Work out the finished part from the listing and answer in its coordinate system (mm). Face numbers are marked on the shaded views. A direction names the side the tool comes from. Coordinates: 2 decimals unless noted, no trailing zeros. Write each loop counter-clockwise with the first axis right and the second up, starting at its lowest first coordinate (ties: lowest second). Pieces come first, ordered by that corner, then holes. Notation, with made-up numbers: M 87,36.25 L 127,36.25 A14 ccw 127,56.25 Z; hole C -35,-14.75 d6. An arc over 180 degrees is marked long. Answer as CSV lines item,"result". Start each with the question number.
(1) Flat-ended cylindrical pins translate along their axes: P1, Ø3.5, axis at x = -243.73, y = 56.34, coming from the -Z side; P2, Ø4, axis at x = -194, z = 7.5, coming from the +Y side; P3, Ø3, axis at x = -229, z = 2.5, coming from the +Y side. Find the tip coordinate at first contact, or state that the pin passes through.
(2) The mould has two halves that part along X. Classify the marked faces 3, 4, 5 and 6: released by +X, released by -X, zero draft, split by the parting line, or undercut.
(3) Find the intervals of material crossed by L1, parallel to X at y = 53, z = 11; L2, parallel to Y at x = -185, z = 6.5; L3, parallel to X at y = 64, z = 8.25, in increasing order. Write a range as [from, to].
(4) For the marked faces 1 and 2, determine the directions among +Z, -Z, +X, -X, +Y, -Y from which every point of the face is accessible in a straight line to the end or side of a thin tool.
(5) A cutting plane is placed at B-B on z = 11. Count the separate pieces of the cut face and the enclosed holes in it, then the cut area to 3 significant figures.
(6) A cutting plane is placed at A-A on y = 2. Give the vertices of the cut face in (x, z).
(7) A cutting plane is placed at C-C on x = -179.5. Give the vertices of the cut face in (y, z).
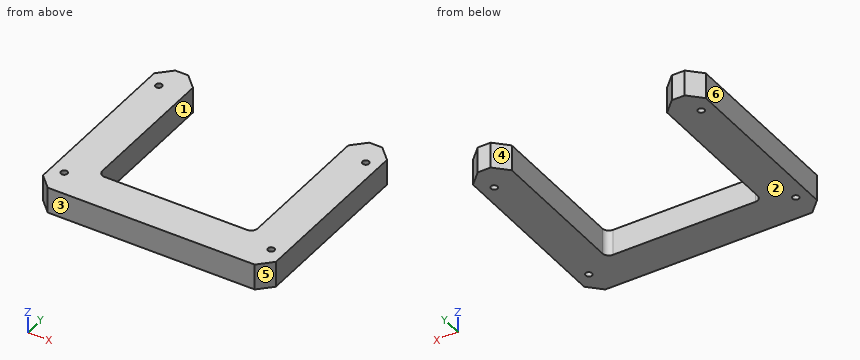
from build123d import *

# Parameters (mm, degrees)
BOSS_EXTRUDE1_DEPTH = 12.7
FILLET1_R           = 3.175
CHAMFER1_SIZE       = 6.35
HOLE1_D             = 3.175
HOLE1_DEPTH         = 31.75
HOLE1_CSINK_D       = 10.16
HOLE1_CSINK_ANGLE   = 82
HOLE1_TIP           = 0.953866233


with BuildPart() as part:
    # Sketch1 → Boss-Extrude1 (new body)
    with BuildSketch(Plane.XY):
        Polygon((-231.027465963, 69.04320968), (-231.027465963, -10.33179032), (-154.827465963, -10.33179032), (-154.827465963, 69.04320968), (-135.777465963, 69.04320968), (-135.777465963, -29.38179032), (-250.077465963, -29.38179032), (-250.077465963, 69.04320968), align=None)
    extrude(amount=BOSS_EXTRUDE1_DEPTH)

    # Fillet1
    fillet1_edges = [part.edges().sort_by_distance(p)[0] for p in [
        (-231.027465963, -10.33179032, 6.35),
        (-154.827465963, -10.33179032, 6.35),
    ]]
    fillet(fillet1_edges, radius=FILLET1_R)

    # Chamfer1
    chamfer1_edges = [part.edges().sort_by_distance(p)[0] for p in [
        (-231.027465963, 69.04320968, 6.35),
        (-154.827465963, 69.04320968, 6.35),
        (-135.777465963, 69.04320968, 6.35),
        (-135.777465963, -29.38179032, 6.35),
        (-250.077465963, -29.38179032, 6.35),
        (-250.077465963, 69.04320968, 6.35),
    ]]
    chamfer(chamfer1_edges, length=CHAMFER1_SIZE)

    # Hole1
    with Locations(Plane(origin=(-124.004465969, -215.287141225, -12.7), x_dir=(-1, 0, 0), z_dir=(0, 0, -1))):
        with Locations((113.649999994, 128.807623392), (113.649999994, 23.940956725), (-94.599999994, 161.374290059), (94.599999994, 161.374290059), (0, 161.374290059), (0, 193.124290059), (0, 440.553783621), (0, 301.970350905), (40.979166666, 301.970350905), (166.795833328, 301.970350905), (207.774999994, 440.553783621), (207.774999994, 333.02141023), (207.774999994, 225.48903684), (207.774999994, 137.424290059), (207.774999994, 10.424290059), (-207.774999994, 10.424290059), (-207.774999994, 137.424290059), (-207.774999994, 225.48903684), (-207.774999994, 333.02141023), (-207.774999994, 440.553783621), (-166.795833328, 301.970350905), (-40.979166666, 301.970350905), (-113.649999994, 23.940956725), (-113.649999994, 128.807623392), (119.722999994, 198.605350905), (119.722999994, 271.630350905), (18.122999994, 198.605350905), (18.122999994, 271.630350905)):
            CounterSinkHole(HOLE1_D / 2, HOLE1_CSINK_D / 2, depth=HOLE1_DEPTH, counter_sink_angle=HOLE1_CSINK_ANGLE)
            with Locations((0, 0, -(HOLE1_DEPTH + HOLE1_TIP / 2))):  # 118° drill point
                Cone(0, HOLE1_D / 2, HOLE1_TIP, mode=Mode.SUBTRACT)


solid = part.part
Here are the results:
1,P1,"stops at z = 0"
1,P2,"stops at y = -10.33"
1,P3,"stops at y = -8.91"
2,face 3,"zero draft"
2,face 4,"undercut"
2,face 5,"released by +X"
2,face 6,"released by -X"
3,L1,"x = [-250.08, -231.03], [-154.83, -135.78]"
3,L2,"y = [-29.38, -10.33]"
3,L3,"x = [-248.77, -232.33], [-153.52, -137.08]"
4,face 1,"+Z, -Z, +Y"
4,face 2,"-Z, +X, -X, +Y, -Y"
5,separate pieces,"1"
5,enclosed holes,"4"
5,area,"5,050 mm^2"
6,outline,"M -250.08,0 L -231.03,0 L -231.03,12.7 L -250.08,12.7 Z; M -154.83,0 L -135.78,0 L -135.78,12.7 L -154.83,12.7 Z"
7,outline,"M -29.38,0 L -10.33,0 L -10.33,12.7 L -29.38,12.7 Z"
